from build123d import *

# Parameters (mm, degrees)
SKETCH_1_W          = 145
SKETCH_1_H          = 155
SKETCH_1_R          = 1.6
EXTRUDE_1_DEPTH     = 5
SKETCH_2_W          = 60
SKETCH_2_H          = 5
EXTRUDE_2_DEPTH     = 20
SKETCH_3_W          = 145
SKETCH_3_H          = 155
SKETCH_3_W_2        = 135
SKETCH_3_H_2        = 145
EXTRUDE_3_DEPTH     = 60
SKETCH_8_R          = 1.6
EXTRUDE_7_DEPTH     = 4.5
SKETCH_9_W          = 76
SKETCH_9_H          = 90
CUT_EXTRUDE_1_DEPTH = 10
CUT_EXTRUDE_2_DEPTH = 3.5
SKETCH_14_R         = 6
CUT_EXTRUDE_3_DEPTH = 10
SKETCH_15_R         = 6
CUT_EXTRUDE_4_DEPTH = 10


with BuildPart() as part:
    # 草图1 → 凸台-拉伸1 (new body)
    with BuildSketch(Plane.XY):
        with Locations((0, -18.75)):
            Rectangle(SKETCH_1_W, SKETCH_1_H)
        with Locations(Location((-61.35, 46.25, 0), (0, 0, 180))):
            Circle(SKETCH_1_R, mode=Mode.SUBTRACT)
        with Locations(Location((61.35, -46.6, 0), (0, 0, 180))):
            Circle(SKETCH_1_R, mode=Mode.SUBTRACT)
        with Locations(Location((61.35, 46.6, 0), (0, 0, 180))):
            Circle(SKETCH_1_R, mode=Mode.SUBTRACT)
        with Locations(Location((-61.35, -46.25, 0), (0, 0, 180))):
            Circle(SKETCH_1_R, mode=Mode.SUBTRACT)
        with Locations(Location((62.35, 31.5, 0), (0, 0, 180))):
            Circle(SKETCH_1_R, mode=Mode.SUBTRACT)
        with Locations(Location((62.35, -23.5, 0), (0, 0, 180))):
            Circle(SKETCH_1_R, mode=Mode.SUBTRACT)
        with Locations(Location((-49.95, 31.5, 0), (0, 0, 180))):
            Circle(SKETCH_1_R, mode=Mode.SUBTRACT)
        with Locations(Location((-49.95, -23.5, 0), (0, 0, 180))):
            Circle(SKETCH_1_R, mode=Mode.SUBTRACT)
    extrude(amount=EXTRUDE_1_DEPTH)

    # 草图2 → 凸台-拉伸2 (add)
    with BuildSketch(Plane.XY.offset(5)):
        with Locations((0, -37.5)):
            Rectangle(SKETCH_2_W, SKETCH_2_H)
        with Locations((0, -82)):
            Rectangle(SKETCH_2_W, SKETCH_2_H)
    extrude(amount=EXTRUDE_2_DEPTH)

    # 草图3 → 凸台-拉伸3 (add)
    with BuildSketch(Plane.XY.offset(5)):
        with Locations((0, -18.75)):
            Rectangle(SKETCH_3_W, SKETCH_3_H)
        with Locations((0, -18.75)):
            Rectangle(SKETCH_3_W_2, SKETCH_3_H_2, mode=Mode.SUBTRACT)
    extrude(amount=EXTRUDE_3_DEPTH)

    # 草图8 → 凸台-拉伸7 (add)
    # profile 1 of 2: a face of its own
    with BuildSketch(Plane.XY.offset(65)):
        Polygon((-67.5, -76.25), (-52.5, -91.25), (-67.5, -91.25), align=None)
        with Locations((-62.5, -86.25)):
            Circle(SKETCH_8_R, mode=Mode.SUBTRACT)
    # profile 2 of 2: a face of its own
    with BuildSketch(Plane.XY.offset(65)):
        Polygon((67.5, -91.25), (52.5, -91.25), (67.5, -76.25), align=None)
        with Locations(Location((62.5, -86.25, 0), (0, 0, 180))):
            Circle(SKETCH_8_R, mode=Mode.SUBTRACT)
    extrude(amount=-EXTRUDE_7_DEPTH)

    # 草图9 → 切除-拉伸1 (cut)
    with BuildSketch(Plane.XZ.offset(-53.75)):
        with Locations((29.5, 76)):
            Rectangle(SKETCH_9_W, SKETCH_9_H)
    extrude(amount=-CUT_EXTRUDE_1_DEPTH, mode=Mode.SUBTRACT)

    # 草图13 → 切除-拉伸2 (cut)
    with BuildSketch(Plane.XY.offset(5)):
        Polygon((-30, -79.5), (-58, -79.5), (-58, -40), (58, -40), (58, -79.5), align=None)
    extrude(amount=-CUT_EXTRUDE_2_DEPTH, mode=Mode.SUBTRACT)

    # 草图14 → 切除-拉伸3 (cut)
    with BuildSketch(Plane(origin=(72.5, 0, 0), x_dir=(0, 0, -1), z_dir=(1, 0, 0))):
        with Locations(Location((-20.643106149, -83.462816737, 0), (0, 0, 90))):
            Circle(SKETCH_14_R)
    extrude(amount=-CUT_EXTRUDE_3_DEPTH, mode=Mode.SUBTRACT)

    # 草图15 → 切除-拉伸4 (cut)
    with BuildSketch(Plane(origin=(0, -96.25, 0), x_dir=(-1, 0, 0), z_dir=(0, -1, 0))):
        with Locations(Location((-30, -30, 0), (0, 0, 180))):
            Circle(SKETCH_15_R)
        with Locations(Location((30, -30, 0), (0, 0, 270))):
            Circle(SKETCH_15_R)
    extrude(amount=-CUT_EXTRUDE_4_DEPTH, mode=Mode.SUBTRACT)


solid = part.part
The model under review builds one solid part; all positions refer to its coordinate system, in mm. A direction names the side the tool comes from. Coordinates: 2 decimals unless noted, no trailing zeros. Write each loop counter-clockwise with the first axis right and the second up, starting at its lowest first coordinate (ties: lowest second). Pieces come first, ordered by that corner, then holes. Notation, with made-up numbers: (49, 5.25) -> (62, 5.25) arc R29 ccw to (62, 31.25) -> close; hole circle Ø6 at (-17, 85.5). An arc over 180 degrees is marked (long way). Answer in a Markdown table with one row per item.
1. We need section A-A, the plane y = 14.5. State the section outline as (x, z) points.
Answers below:
| item | result |
|---|---|
| outline | (-72.5, 0) -> (72.5, 0) -> (72.5, 65) -> (67.5, 65) -> (67.5, 5) -> (-67.5, 5) -> (-67.5, 65) -> (-72.5, 65) -> close |
2. Clearance check with flat-ended pins moving along their axes: pin 1 Ø1.9 at (x, y) = (62.5, -86.25) entering from +Z; pin 2 Ø3 at (x, y) = (-49.95, -23.5) entering from -Z; pin 3 Ø5.5 at (x, y) = (7.5, -82) entering from +Z; pin 4 Ø1.5 at (x, y) = (40.5, 57.5) entering from +Z. State where each tip first meets the part, or that it passes through.
Answers below:
| item | result |
|---|---|
| pin 1 | stops at z = 5 |
| pin 2 | passes through |
| pin 3 | stops at z = 25 |
| pin 4 | stops at z = 31 |
3. We need section C-C, the plane x = 46. State the section outline as (y, z) points.
Answers below:
| item | result |
|---|---|
| outline | (-96.25, 0) -> (58.75, 0) -> (58.75, 31) -> (53.75, 31) -> (53.75, 5) -> (-40, 5) -> (-40, 1.5) -> (-79.5, 1.5) -> (-79.5, 5) -> (-91.25, 5) -> (-91.25, 65) -> (-96.25, 65) -> close |
4. Draft analysis for pull direction X (two halves, no side actions). For faces 6 (the flat face through (-1, -79.5, 13)), 7 (the flat face through (-1, -40, 13)), 8 (the flat face through (72.5, -20, 32)), 9 (the flat face through (-1, -18, 0)), state which applies: +X half, -X half, draft (parallel to the pull), parting line (faces both ways), or undercut.
Answers below:
| item | result |
|---|---|
| face 6 | undercut |
| face 7 | undercut |
| face 8 | +X half |
| face 9 | draft |
5. Wall thickness on probe 1 along Y at (x, z) = (-49.95, 1.85); probe 2 along X at (y, z) = (46.25, 1.45); probe 3 along X at (y, z) = (-76, 53): over which ranges is each line inside the solid? List them lowest first. Write a range as [from, to].
Answers below:
| item | result |
|---|---|
| probe 1 | y = [-96.25, -79.5], [-40, -25.1], [-21.9, 29.9], [33.1, 58.75] |
| probe 2 | x = [-72.5, -62.95], [-59.75, 59.79], [62.91, 72.5] |
| probe 3 | x = [-72.5, -67.5], [67.5, 72.5] |
6. For faces 1 (the cylindrical face through (70.04, -77.74, 22.45)), 2 (the flat face through (65, -87, 60.5)), 3 (the cylindrical face through (28.699, -93.785, 24.143)), 4 (the flat face through (-58, -60, 3)), 5 (the flat face through (59.895, -83.855, 62.782)), list the 3-axis set-ups (+Z, -Z, +X, -X, +Y, -Y) from which the entire face can be reached by the end or side of a thin tool; tool diameter is ignored.
Answers below:
| item | result |
|---|---|
| face 1 | +X |
| face 2 | +Y |
| face 3 | -Y |
| face 4 | +Z |
| face 5 | +Z, +Y |
7. We need section B-B, the plane z = 47.5. State the section outline as (x, y) points.
Answers below:
| item | result |
|---|---|
| outline | (-72.5, -96.25) -> (72.5, -96.25) -> (72.5, 58.75) -> (67.5, 58.75) -> (67.5, -91.25) -> (-67.5, -91.25) -> (-67.5, 53.75) -> (-8.5, 53.75) -> (-8.5, 58.75) -> (-72.5, 58.75) -> close |
